Design review of the part built by this model. Coordinates are the model's own, in mm. Coordinates: 2 decimals unless noted, no trailing zeros. Write each loop counter-clockwise with the first axis right and the second up, starting at its lowest first coordinate (ties: lowest second). Pieces come first, ordered by that corner, then holes.
Q1. Mouldability with a two-part tool opening along X and no side actions: class faces 1 (the flat face through (1, 0, 0)), 2 (the cylindrical face through (-2.5, -4.9, 5.1)), 3 (the flat face through (30, 0, 5)), 4 (the flat face through (-30, 0, 5)) as pulls with the +X half, pulls with the -X half, needs draft (parallel to the pull), parting line crosses it, or undercut.
Q2. Take a section at D-D (x = -25). Give the boundary of the cut face in (y, z), and give its area (3 significant figures).
Q3. Take a section at A-A (x = -5). Give the boundary of the cut face in (y, z).
Q4. Take a section at C-C (z = 5). Give the boundary of the cut face in (x, y), and give its area (3 significant figures).
Q5. For probe 1 along Y at (x, z) = (-5, 3.75); probe 2 along X at (y, z) = (1, 0.5); probe 3 along X at (y, z) = (1, 4), list the stretches that pass through material, from the lowest coordinate up.
Q6. Take a section at B-B (y = 0). Give the boundary of the cut face in (x, z), and give its area (3 significant figures).
```python
from build123d import *

# Parameters (mm, degrees)
SKETCH_1_W          = 60
SKETCH_1_H          = 50
EXTRUDE_1_DEPTH     = 10
SKETCH_2_R          = 5.5
CUT_EXTRUDE_1_DEPTH = 10
FILLET_1_R          = 3


with BuildPart() as part:
    # 草图1 → 凸台-拉伸1 (new body)
    with BuildSketch(Plane.XY):
        Rectangle(SKETCH_1_W, SKETCH_1_H)
    extrude(amount=EXTRUDE_1_DEPTH)

    # 草图2 → 切除-拉伸1 (cut)
    with BuildSketch(Plane.XY.offset(10)):
        with Locations((-5, 0)):
            Circle(SKETCH_2_R)
    extrude(amount=-CUT_EXTRUDE_1_DEPTH, mode=Mode.SUBTRACT)

    # 圆角1
    fillet_1_edges = [part.edges().sort_by_distance(p)[0] for p in [
        (-30, 0, 10),
        (0, -25, 10),
        (0, -25, 0),
        (-30, 0, 0),
        (0, 25, 0),
        (0, 25, 10),
    ]]
    fillet(fillet_1_edges, radius=FILLET_1_R)


solid = part.part
```
Response:
1. face 1: needs draft
1. face 2: undercut
1. face 3: pulls with the +X half
1. face 4: pulls with the -X half
2. outline: (-25, 3) arc R3 ccw to (-22, 0) - (22, 0) arc R3 ccw to (25, 3) - (25, 7) arc R3 ccw to (22, 10) - (-22, 10) arc R3 ccw to (-25, 7) - close
2. area: 492 mm2
3. outline: (-25, 3) arc R3 ccw to (-22, 0) - (-5.5, 0) - (-5.5, 10) - (-22, 10) arc R3 ccw to (-25, 7) - close; (5.5, 0) - (22, 0) arc R3 ccw to (25, 3) - (25, 7) arc R3 ccw to (22, 10) - (5.5, 10) - close
4. outline: (-30, -25) - (30, -25) - (30, 25) - (-30, 25) - close; hole circle Ø11 at (-5, 0)
4. area: 2,900 mm2
5. probe 1: y = -25 to -5.5, 5.5 to 25
5. probe 2: x = -28.66 to -10.41, 0.41 to 30
5. probe 3: x = -30 to -10.41, 0.41 to 30
6. outline: (-30, 3) arc R3 ccw to (-27, 0) - (-10.5, 0) - (-10.5, 10) - (-27, 10) arc R3 ccw to (-30, 7) - close; (0.5, 0) - (30, 0) - (30, 10) - (0.5, 10) - close
6. area: 486 mm2
